Source: CAD feature listing. Evaluate the final solid. Frame: model axes, mm. A direction names the side the tool comes from. Coordinates: 2 decimals unless noted, no trailing zeros. Write each loop counter-clockwise with the first axis right and the second up, starting at its lowest first coordinate (ties: lowest second). Pieces come first, ordered by that corner, then holes. Notation, with made-up numbers: (44.5, -21.5) -> (90.5, -21.5) arc R7 cw to (90.5, -9.5) -> close; hole circle Ø7 at (69, 33.25). An arc over 180 degrees is marked (long way). One line per item, written item: value. Start each with the question number.
1. Section query B-B, the plane z = -1.35. Output: boundary loops of the cut face in (x, y) (3 decimals), and give its area (3 significant figures).
2. Line query: line 1 (X direction, y = 0.1, z = -2); line 2 (X direction, y = 0.95, z = -2.4); line 3 (Y direction, x = 18.5, z = -1.95) (3 decimals). Output: solid intervals per line, ascending.
3. First-contact query: P1, Ø1.9, axis at x = 1.651, z = -1.651, coming from the +Y side (3 decimals). Flat tip, straight axial feed; report the tip coordinate or a pass-through.
4. Mould query, pull axis Z, two halves, no side actions, for faces 3 (the flat face through (9, 1, -3.302)), 4 (the flat face through (9, 1, 0)), 5 (the cylindrical face through (0.89, 0.31, -1.33)). Classes: released by +Z, released by -Z, zero draft, split by the parting line, or undercut.
5. Access query for faces 1 (the flat face through (0, 1, -2)), 2 (the cylindrical face through (16.167, 0.957, -1.14)). Directions: +Z, -Z, +X, -X, +Y, -Y. A direction counts if a zero-diameter tool reaches every point of the face in a straight line with its end or side. Return the directions, or none.
6. Section query C-C, the plane y = 1. Output: boundary loops of the cut face in (x, z).
7. Section query D-D, the plane z = -0.5. Output: boundary loops of the cut face in (x, y) (3 decimals), and give its area (3 significant figures).
8. Section query A-A, the plane x = 17. Output: boundary loops of the cut face in (y, z) (3 decimals).
from build123d import *

# Parameters (mm, degrees)
SKETCH1_W                                           = 19.05
SKETCH1_H                                           = 3.302
BOSS_EXTRUDE1_DEPTH                                 = 1.27
CBORE_FOR_00_BINDING_HEAD_MACHINE_SCREW_D           = 1.651
CBORE_FOR_00_BINDING_HEAD_MACHINE_SCREW_CBORE_D     = 2.667
CBORE_FOR_00_BINDING_HEAD_MACHINE_SCREW_CBORE_DEPTH = 0.635


with BuildPart() as part:
    # Sketch1 → Boss-Extrude1 (new body)
    with BuildSketch(Plane(origin=(0, 0, 0), x_dir=(1, 0, 0), z_dir=(0, 1, 0))):
        with Locations((9.525, 1.651)):
            Rectangle(SKETCH1_W, SKETCH1_H)
    extrude(amount=BOSS_EXTRUDE1_DEPTH)

    # CBORE for #00 Binding Head Machine Screw1 (through all)
    with Locations(Plane(origin=(0, 1.27, 0), x_dir=(1, 0, 0), z_dir=(0, 1, 0))):
        with Locations((1.651, 1.651)):
            cbore_for_00_binding_head_machine_screw = CounterBoreHole(CBORE_FOR_00_BINDING_HEAD_MACHINE_SCREW_D / 2, CBORE_FOR_00_BINDING_HEAD_MACHINE_SCREW_CBORE_D / 2, CBORE_FOR_00_BINDING_HEAD_MACHINE_SCREW_CBORE_DEPTH)

    # Mirror1: CBORE for #00 Binding Head Machine Screw1 across plane
    add(cbore_for_00_binding_head_machine_screw.mirror(Plane.ZY.offset(-9.525)), mode=Mode.SUBTRACT)


solid = part.part
Computed values:
1. outline: (0, 0) -> (0.882, 0) -> (0.882, 0.635) -> (0.352, 0.635) -> (0.352, 1.27) -> (0, 1.27) -> close; (2.42, 0) -> (16.63, 0) -> (16.63, 0.635) -> (16.1, 0.635) -> (16.1, 1.27) -> (2.95, 1.27) -> (2.95, 0.635) -> (2.42, 0.635) -> close; (18.168, 0) -> (19.05, 0) -> (19.05, 1.27) -> (18.698, 1.27) -> (18.698, 0.635) -> (18.168, 0.635) -> close
1. area: 18.9 mm²
2. line 1: x = 0 to 0.9, 2.4 to 16.65, 18.15 to 19.05
2. line 2: x = 0 to 0.55, 2.75 to 16.3, 18.5 to 19.05
2. line 3: y = 0 to 0.635
3. P1: stops at y = 0.635
4. face 3: released by -Z
4. face 4: released by +Z
4. face 5: undercut
5. face 1: +Z, -Z, -X, +Y, -Y
5. face 2: +Y
6. outline: (0, -3.3) -> (19.05, -3.3) -> (19.05, 0) -> (0, 0) -> close; hole circle Ø2.67 at (1.65, -1.65); hole circle Ø2.67 at (17.4, -1.65)
7. outline: (0, 0) -> (19.05, 0) -> (19.05, 1.27) -> (18.072, 1.27) -> (18.072, 0.635) -> (16.726, 0.635) -> (16.726, 1.27) -> (2.324, 1.27) -> (2.324, 0.635) -> (0.978, 0.635) -> (0.978, 1.27) -> (0, 1.27) -> close
7. area: 22.5 mm²
8. outline: (0, -3.302) -> (1.27, -3.302) -> (1.27, -2.923) -> (0.635, -2.923) -> (0.635, -2.374) -> (0, -2.374) -> close; (0, -0.928) -> (0.635, -0.928) -> (0.635, -0.379) -> (1.27, -0.379) -> (1.27, 0) -> (0, 0) -> close
